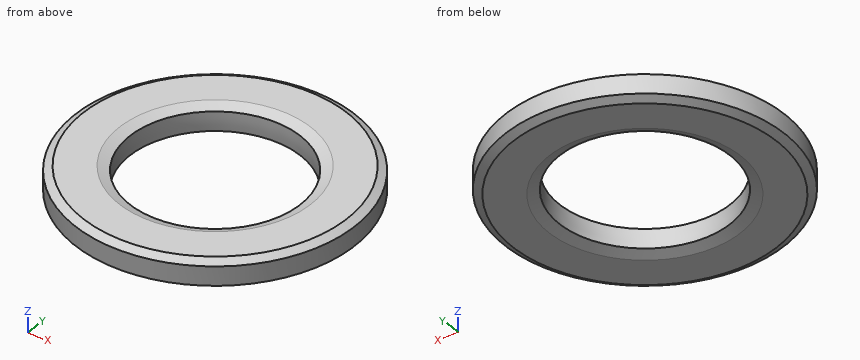
```python
from build123d import *
from OCP.BRepFilletAPI import BRepFilletAPI_MakeChamfer

# Parameters (mm, degrees)
BOSS_EXTRUDE1_DEPTH      = 0.79375
BOSS_EXTRUDE1_DEPTH_BACK = 0.79375
SKETCH3_R                = 7.9375
SKETCH3_R_2              = 4.826
CHAMFER1_SIZE            = 0.254
CHAMFER1_SIZE2           = 0.439940905
CHAMFER2_SIZE            = 0.570578725


with BuildPart() as part:
    # Sketch3 → Boss-Extrude1 (new, two sides: drawn at the far end of the back side and taken through both)
    with BuildSketch(Plane.XY.offset(-BOSS_EXTRUDE1_DEPTH_BACK)):
        Circle(SKETCH3_R)
        Circle(SKETCH3_R_2, mode=Mode.SUBTRACT)
    extrude(amount=BOSS_EXTRUDE1_DEPTH + BOSS_EXTRUDE1_DEPTH_BACK)

    # Chamfer1: one chamfer whose edges measure the first distance from different faces: ONE call of the kernel's chamfer builder (chamfer() names one face for all edges)
    chamfer1_edges_1 = [part.edges().sort_by_distance(p)[0] for p in [
        (-7.9375, 0, 0.79375),
    ]]
    chamfer1_side_1 = [part.faces().sort_by_distance(p)[0] for p in [
        (-7.9375, 0, 0.396875),
    ]]
    chamfer1_edges_2 = [part.edges().sort_by_distance(p)[0] for p in [
        (-7.9375, 0, -0.79375),
    ]]
    chamfer1_side_2 = [part.faces().sort_by_distance(p)[0] for p in [
        (-7.9375, 0, -0.396875),
    ]]
    chamfer1 = BRepFilletAPI_MakeChamfer(part.part.solid().wrapped)
    for e in chamfer1_edges_1:
        chamfer1.Add(CHAMFER1_SIZE, CHAMFER1_SIZE2, e.wrapped, chamfer1_side_1[0].wrapped)  # the first distance lies on this face
    for e in chamfer1_edges_2:
        chamfer1.Add(CHAMFER1_SIZE, CHAMFER1_SIZE2, e.wrapped, chamfer1_side_2[0].wrapped)  # the first distance lies on this face
    add(Compound.cast(chamfer1.Shape()), mode=Mode.REPLACE)

    # Sketch4 → Cut-Revolve1 (revolve, cut)
    with BuildSketch(Plane(origin=(0, 0, 0), x_dir=(0, 0, -1), z_dir=(1, 0, 0)), mode=Mode.PRIVATE) as cut_revolve1_sk:
        with BuildLine():
            Line((-0.79375, 4.7752), (-0.79375, 4.8768))
            ThreePointArc((-0.79375, 4.8768), (0, 4.826), (0.79375, 4.8768))
            Line((0.79375, 4.8768), (0.79375, 4.7752))
            Line((0.79375, 4.7752), (-0.79375, 4.7752))
        make_face()
    revolve(cut_revolve1_sk.sketch.rotate(Axis((0, 0, 0.79375), (0, 0, -1)), 90), axis=Axis((0, 0, 0.79375), (0, 0, -1)), mode=Mode.SUBTRACT)

    # Chamfer2
    # the kernel refuses this chamfer: 0.570578725, 0.254 mm, written as the material it takes off along each edge
    with BuildSketch(Plane(origin=(0, 0, -0.79375), x_dir=(1, 0, 0), z_dir=(0, 1, 0))) as chamfer2_piece_1:
        with BuildLine():
            Line((4.8768 + CHAMFER2_SIZE, 0), (4.849816205, -0.249673341))
            ThreePointArc((4.849816205, -0.249673341), (4.86146095, -0.130166676), (4.8768, 0))
            Line((4.8768, 0), (4.8768 + CHAMFER2_SIZE, 0))
        make_face()
    revolve(axis=Axis((0, 0, -0.79375), (0, 0, -1)), mode=Mode.SUBTRACT)
    with BuildSketch(Plane(origin=(0, 0, 0.79375), x_dir=(1, 0, 0), z_dir=(0, 1, 0))) as chamfer2_piece_2:
        with BuildLine():
            Line((4.8768 + CHAMFER2_SIZE, 0), (4.849816205, 0.249673341))
            ThreePointArc((4.849816205, 0.249673341), (4.86146095, 0.130166676), (4.8768, 0))
            Line((4.8768, 0), (4.8768 + CHAMFER2_SIZE, 0))
        make_face()
    revolve(axis=Axis((0, 0, 0.79375), (0, 0, -1)), mode=Mode.SUBTRACT)


solid = part.part
```
The model under review builds one solid part; all positions refer to its coordinate system, in mm. Round coordinates to 2 decimals unless told otherwise and drop trailing zeros. Loops run counter-clockwise (first coordinate to the right, second up) from the corner with the lowest first, then second, coordinate; pieces in that order, holes last.
1) Consider section A-A on x = 0. State the section outline as (y, z) points, then the cut area to 3 significant figures.
Values follow:
outline: (-7.94, -0.54) - (-7.5, -0.79) - (-5.45, -0.79) - (-4.85, -0.54) arc R6.23 ccw to (-4.85, 0.54) - (-5.45, 0.79) - (-7.5, 0.79) - (-7.94, 0.54) - close; (4.85, -0.54) - (5.45, -0.79) - (7.5, -0.79) - (7.94, -0.54) - (7.94, 0.54) - (7.5, 0.79) - (5.45, 0.79) - (4.85, 0.54) arc R6.23 ccw to start
area: 9.32 mm2
2) Consider section C-C on z = 0.35. State the section outline as (x, y) points (1 decimal), then the cut area to 3 significant figures.
Values follow:
outline: circle Ø15.9 at (0, 0); hole circle Ø9.7 at (0, 0)
area: 124 mm2
3) Wall thickness on line 1 along X through (y, z) = (3.25, 0.5); line 2 along X through (y, z) = (0.5, 0.1); line 3 along Y through (x, z) = (-3.25, 0.05): over which ranges is each line inside the solid? List them lowest first.
Values follow:
line 1: x = -7.24 to -3.59, 3.59 to 7.24
line 2: x = -7.92 to -4.8, 4.8 to 7.92
line 3: y = -7.24 to -3.57, 3.57 to 7.24
